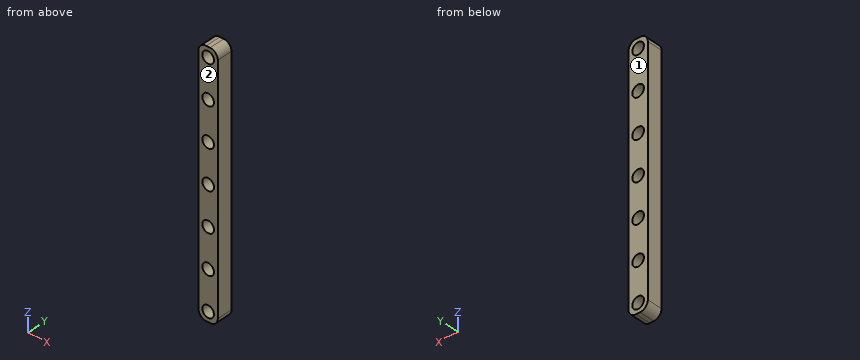
```python
from build123d import *

# Parameters (mm, degrees)
SKETCH2_W           = 5
SKETCH2_H           = 65
BOSS_EXTRUDE1_DEPTH = 4
SKETCH3_R           = 1.5
CUT_EXTRUDE1_DEPTH  = 4
FILLET2_R           = 2


with BuildPart() as part:
    # Sketch2 → Boss-Extrude1 (new body)
    with BuildSketch(Plane(origin=(0, 0, 0), x_dir=(1, 0, 0), z_dir=(0, 1, 0))):
        with Locations((-2.5, 32.5)):
            Rectangle(SKETCH2_W, SKETCH2_H)
    extrude(amount=BOSS_EXTRUDE1_DEPTH)

    # Sketch3 → Cut-Extrude1 (cut)
    with BuildSketch(Plane(origin=(0, 4, 0), x_dir=(1, 0, 0), z_dir=(0, 1, 0))):
        with Locations((-2.5, 32.5)):
            Circle(SKETCH3_R)
        with Locations((-2.5, 22.5)):
            Circle(SKETCH3_R)
        with Locations((-2.5, 12.5)):
            Circle(SKETCH3_R)
        with Locations((-2.5, 2.5)):
            Circle(SKETCH3_R)
        with Locations((-2.5, 42.5)):
            Circle(SKETCH3_R)
        with Locations((-2.5, 52.5)):
            Circle(SKETCH3_R)
        with Locations((-2.5, 62.5)):
            Circle(SKETCH3_R)
    extrude(amount=-CUT_EXTRUDE1_DEPTH, mode=Mode.SUBTRACT)

    # Fillet2
    fillet2_edges = [part.edges().sort_by_distance(p)[0] for p in [
        (0, 2, 0),
        (0, 2, -65),
        (-5, 2, -65),
        (-5, 2, 0),
    ]]
    fillet(fillet2_edges, radius=FILLET2_R)


solid = part.part
```
Build history of the part. All positions in model axes, mm. Face numbers are marked on the shaded views. Give positions to 0.01 mm unless a question says otherwise; leave off trailing zeros. Order: outer loops, then holes, each group sorted by start corner. A loop starts at its lowest first (then second) coordinate and runs counter-clockwise, first axis right, second up. Notation, with made-up numbers: M -7,24.25 L 45,24.25 A30 ccw 45,57.25 Z; hole C 85,-3 d3. An arc over 180 degrees is marked long. Write item = value, one per line. Start each with the question number.
(1) Slice it at A-A on z = -22.5. Write the cut outline in (x, y).
(2) Probe L1, parallel to X at y = 0.95, z = -12.5; L2, parallel to X at y = 0.9, z = -11.5; L3, parallel to Z at x = -0.65, y = 2.5. List the from-to ranges inside material, lowest first. Write a range as [from, to].
(3) Two-plate mould, pull along Y, no slides. Class the marked faces 1 and 2: released by +Y, released by -Y, zero draft, split by the parting line, or undercut.
(4) Slice it at B-B on y = 0.8. Write the cut outline in (x, z), plus the area to 3 significant figures.
Responses:
q1.outline = M -5,0 L -4,0 L -4,4 L -5,4 Z; M -1,0 L 0,0 L 0,4 L -1,4 Z
q2.L1 = [-5, -4], [-1, 0]
q2.L2 = [-5, -3.62], [-1.38, 0]
q2.L3 = [-64.48, -0.52]
q3.face_1 = released by +Y
q3.face_2 = released by -Y
q4.outline = M -5,-63 A2 ccw -3,-65 L -2,-65 A2 ccw 0,-63 L 0,-2 A2 ccw -2,0 L -3,0 A2 ccw -5,-2 Z; hole C -2.5,-62.5 d3; hole C -2.5,-52.5 d3; hole C -2.5,-42.5 d3; hole C -2.5,-32.5 d3; hole C -2.5,-22.5 d3; hole C -2.5,-12.5 d3; hole C -2.5,-2.5 d3
q4.area = 272 mm2
